```python
from build123d import *

# Parameters (mm, degrees)
SKETCH1_R                                 = 36.5125
SKETCH1_R_2                               = 19.05
EXTRUDE1_DEPTH                            = 44.45
SKETCH3_R                                 = 22.6187
OUTER_RACE_POCKET_MASTER_DEPTH            = 15.9258
F_1_4_20_THREAD_PATTERN_MASTER_AT_2_COUNT = 2
F_1_4_20_THREAD_PATTERN_MASTER_AT_2_PITCH = 44.901280605
F_1_4_20_THREAD_PATTERN_MASTER_AT_3_COUNT = 2
F_1_4_20_THREAD_PATTERN_MASTER_AT_3_PITCH = 63.5
F_1_4_20_THREAD_PATTERN_MASTER_AT_4_COUNT = 2
F_1_4_20_THREAD_PATTERN_MASTER_AT_4_PITCH = 44.901280605


with BuildPart() as part:
    # Sketch1 → Extrude1 (new, symmetric)
    with BuildSketch(Plane.XY):
        Circle(SKETCH1_R)
        Circle(SKETCH1_R_2, mode=Mode.SUBTRACT)
    extrude(amount=EXTRUDE1_DEPTH, both=True)

    # Sketch3 → Outer race pocket master (cut)
    with BuildSketch(Plane.XY.offset(44.45)):
        Circle(SKETCH3_R)
    outer_race_pocket_master = extrude(amount=-OUTER_RACE_POCKET_MASTER_DEPTH, mode=Mode.SUBTRACT)

    # Sketch8 → 1/4-20 thread pattern master (revolve, cut)
    with BuildSketch(Plane(origin=(0, 31.75, 44.45), x_dir=(0, -1, 0), z_dir=(1, 0, 0))):
        Polygon((0, 0), (0, 11.058816902), (2.5527, 9.525), (2.5527, 0), align=None)
    f_1_4_20_thread_pattern_master = revolve(axis=Axis((0, 31.75, 50.8), (0, 0, -1)), mode=Mode.SUBTRACT)

    # 1/4-20 thread pattern master at 2: 1/4-20 thread pattern master ×2
    with Locations(*[Vector(0.7071067811865476, -0.7071067811865476, 0) * (i * F_1_4_20_THREAD_PATTERN_MASTER_AT_2_PITCH) for i in range(1, F_1_4_20_THREAD_PATTERN_MASTER_AT_2_COUNT)]):
        add(f_1_4_20_thread_pattern_master, mode=Mode.SUBTRACT)

    # 1/4-20 thread pattern master at 3: 1/4-20 thread pattern master ×2
    with Locations(*[(0, -i * F_1_4_20_THREAD_PATTERN_MASTER_AT_3_PITCH, 0) for i in range(1, F_1_4_20_THREAD_PATTERN_MASTER_AT_3_COUNT)]):
        add(f_1_4_20_thread_pattern_master, mode=Mode.SUBTRACT)

    # 1/4-20 thread pattern master at 4: 1/4-20 thread pattern master ×2
    with Locations(*[Vector(-0.7071067811865476, -0.7071067811865476, 0) * (i * F_1_4_20_THREAD_PATTERN_MASTER_AT_4_PITCH) for i in range(1, F_1_4_20_THREAD_PATTERN_MASTER_AT_4_COUNT)]):
        add(f_1_4_20_thread_pattern_master, mode=Mode.SUBTRACT)

    # Pocket and thread mirror: Outer race pocket master, 1/4-20 thread pattern master across plane
    add(outer_race_pocket_master.mirror(Plane.XY), mode=Mode.SUBTRACT)
    add(f_1_4_20_thread_pattern_master.mirror(Plane.XY), mode=Mode.SUBTRACT)

    # Pocket and thread mirror copy 1 sketch → Pocket and thread mirror copy 1 (revolve, cut)
    with BuildSketch(Plane(origin=(31.75, 0, -44.45), x_dir=(0, -1, 0), z_dir=(1, 0, 0))):
        Polygon((0, 0), (0, -11.058816902), (2.5527, -9.525), (2.5527, 0), align=None)
    revolve(axis=Axis((31.75, 0, -50.8), (0, 0, -1)), mode=Mode.SUBTRACT)

    # Pocket and thread mirror copy 2 sketch → Pocket and thread mirror copy 2 (revolve, cut)
    with BuildSketch(Plane(origin=(0, -31.75, -44.45), x_dir=(0, -1, 0), z_dir=(1, 0, 0))):
        Polygon((0, 0), (0, -11.058816902), (2.5527, -9.525), (2.5527, 0), align=None)
    revolve(axis=Axis((0, -31.75, -50.8), (0, 0, -1)), mode=Mode.SUBTRACT)

    # Pocket and thread mirror copy 3 sketch → Pocket and thread mirror copy 3 (revolve, cut)
    with BuildSketch(Plane(origin=(-31.75, 0, -44.45), x_dir=(0, -1, 0), z_dir=(1, 0, 0))):
        Polygon((0, 0), (0, -11.058816902), (2.5527, -9.525), (2.5527, 0), align=None)
    revolve(axis=Axis((-31.75, 0, -50.8), (0, 0, -1)), mode=Mode.SUBTRACT)


solid = part.part
```
Read the model definition and answer for the solid it produces. Units are mm, in the model's axes. A direction names the side the tool comes from. Give positions to 0.01 mm unless a question says otherwise; leave off trailing zeros. Order: outer loops, then holes, each group sorted by start corner. A loop starts at its lowest first (then second) coordinate and runs counter-clockwise, first axis right, second up.
(1) For faces 4 (the cylindrical face through (-15.12, -11.59, -0.4)), 5 (the cylindrical face through (-0.767, 29.315, -39.754)), 6 (the cylindrical face through (-0.767, 29.315, 39.754)), determine the directions among +Z, -Z, +X, -X, +Y, -Y from which every point of the face is accessible in a straight line to the end or side of a thin tool.
(2) Find section D-D (x = 21). Give the vertices of the cut face in (y, z), plus the area to 3 significant figures.
(3) Find section A-A (y = 8). Give the vertices of the cut face in (x, z).
(4) Find section B-B (x = -11.5). Give the vertices of the cut face in (y, z).
(5) For a pull along X with two mould halves and no side action, classify faces 1 (the conical face through (-31.769, 0.443, 33.658)), 2 (the flat face through (-17, -16, 44.45)), 3 (the cylindrical face through (-0.767, -34.185, 39.754)) as released by +X, released by -X, zero draft, split by the parting line, or undercut.
(6) Given pin 1 (4 mm diameter, centred on x = 31.75, y = 0, fed in from +Z); pin 2 (1 mm diameter, centred on x = 21, z = -20.5, fed in from +Y); pin 3 (4.5 mm diameter, centred on x = 0, y = -31.75, fed in from -Z), each flat-ended and moving along its own axis, determine where each tip first touches the part or whether it passes through.
(7) Straight lines are drawn through the part: L1, parallel to Y at x = 0, z = -39; L2, parallel to Y at x = 0, z = 16; L3, parallel to X at y = -31.75, z = -41.5. For each, find the intervals that lie inside material, in ascending order.
Result sheet:
1. face 4: +Z, -Z
1. face 5: -Z
1. face 6: +Z
2. outline: (-29.87, -44.45) - (-8.4, -44.45) - (-8.4, -28.52) - (8.4, -28.52) - (8.4, -44.45) - (29.87, -44.45) - (29.87, 44.45) - (8.4, 44.45) - (8.4, 28.52) - (-8.4, 28.52) - (-8.4, 44.45) - (-29.87, 44.45) - close
2. area: 4,780 mm2
3. outline: (-35.63, -44.45) - (-21.16, -44.45) - (-21.16, -28.52) - (-17.29, -28.52) - (-17.29, 28.52) - (-21.16, 28.52) - (-21.16, 44.45) - (-35.63, 44.45) - close; (17.29, -28.52) - (21.16, -28.52) - (21.16, -44.45) - (35.63, -44.45) - (35.63, 44.45) - (21.16, 44.45) - (21.16, 28.52) - (17.29, 28.52) - close
4. outline: (-34.65, -44.45) - (-19.48, -44.45) - (-19.48, -28.52) - (-15.19, -28.52) - (-15.19, 28.52) - (-19.48, 28.52) - (-19.48, 44.45) - (-34.65, 44.45) - close; (15.19, -28.52) - (19.48, -28.52) - (19.48, -44.45) - (34.65, -44.45) - (34.65, 44.45) - (19.48, 44.45) - (19.48, 28.52) - (15.19, 28.52) - close
5. face 1: undercut
5. face 2: zero draft
5. face 3: undercut
6. pin 1: stops at z = 34.59
6. pin 2: stops at y = 30.21
6. pin 3: stops at z = -34.74
7. L1: y = -36.51 to -34.3, -29.2 to -22.62, 22.62 to 29.2, 34.3 to 36.51
7. L2: y = -36.51 to -19.05, 19.05 to 36.51
7. L3: x = -18.03 to -2.55, 2.55 to 18.03
